from build123d import *

# Parameters (mm, degrees)
SKETCH_1_W          = 16
SKETCH_1_H          = 16
EXTRUDE_1_DEPTH     = 20
SKETCH_2_W          = 24
SKETCH_2_H          = 24
EXTRUDE_4_DEPTH     = 10
SKETCH_3_W          = 4
SKETCH_3_H          = 3
EXTRUDE_6_DEPTH     = 24
SKETCH_5_R          = 1.6
CUT_EXTRUDE_1_DEPTH = 24
CUT_EXTRUDE_2_DEPTH = 24


with BuildPart() as part:
    # 草图1 → 凸台-拉伸1 (new body)
    with BuildSketch(Plane(origin=(0, 0, 0), x_dir=(1, 0, 0), z_dir=(0, 1, 0))):
        Polygon((-4, 20), (-4, 16), (-4, -4), (16, -4), (20, -4), (20, 0), (20, 20), (0, 20), align=None)
        with Locations((8, 8)):
            Rectangle(SKETCH_1_W, SKETCH_1_H, mode=Mode.SUBTRACT)
    extrude(amount=-EXTRUDE_1_DEPTH)

    # 草图2 → 凸台-拉伸4 (add)
    with BuildSketch(Plane.XZ.offset(20)):
        with Locations((8, -8)):
            Rectangle(SKETCH_2_W, SKETCH_2_H)
    extrude(amount=EXTRUDE_4_DEPTH)

    # 草图3 → 凸台-拉伸6 (add)
    with BuildSketch(Plane.ZY.offset(4)):
        with Locations((10, -36.5)):
            Rectangle(SKETCH_3_W, SKETCH_3_H)
        with BuildLine():
            Line((4, -35), (4, -30))
            Line((4, -30), (-8.000000062, -30))
            ThreePointArc((-8.000000062, -30), (-2.343145773, -32.343145728), (0, -38))
            Line((0, -38), (8, -38))
            Line((8, -38), (8, -35))
            Line((8, -35), (4, -35))
        make_face()
        with BuildLine():
            ThreePointArc((-16, -38), (-13.656854272, -32.343145773), (-8.000000062, -30))
            Line((-8.000000062, -30), (-20, -30))
            Line((-20, -30), (-20, -35))
            Line((-20, -35), (-24, -35))
            Line((-24, -35), (-24, -38))
            Line((-24, -38), (-16, -38))
        make_face()
        with Locations((-26, -36.5)):
            Rectangle(SKETCH_3_W, SKETCH_3_H)
    extrude(amount=-EXTRUDE_6_DEPTH)

    # 草图5 → 切除-拉伸1 (cut)
    with BuildSketch(Plane.XZ.offset(38)):
        with Locations(Location((8, 9, 0), (0, 0, 270))):
            Circle(SKETCH_5_R)
        with Locations(Location((16, 9, 0), (0, 0, 270))):
            Circle(SKETCH_5_R)
        with Locations(Location((0, 9, 0), (0, 0, 90))):
            Circle(SKETCH_5_R)
        with Locations(Location((0, -25, 0), (0, 0, 270))):
            Circle(SKETCH_5_R)
        with Locations(Location((8, -25, 0), (0, 0, 270))):
            Circle(SKETCH_5_R)
        with Locations(Location((16, -25, 0), (0, 0, 270))):
            Circle(SKETCH_5_R)
    extrude(amount=-CUT_EXTRUDE_1_DEPTH, mode=Mode.SUBTRACT)

    # 草图6 → 切除-拉伸2 (cut)
    with BuildSketch(Plane.ZY.offset(4)):
        with BuildLine():
            Line((-20, -35), (-20, 0))
            Line((-20, 0), (4, 0))
            Line((4, 0), (4, -35))
            ThreePointArc((4, -35), (-8, -25.630683123), (-20, -35))
        make_face()
    extrude(amount=-CUT_EXTRUDE_2_DEPTH, mode=Mode.SUBTRACT)


solid = part.part
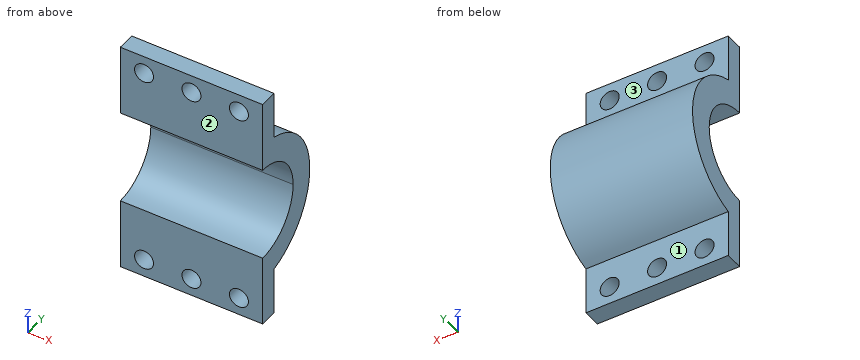
Work out the finished part from the listing and answer in its coordinate system (mm). Face numbers are marked on the shaded views. A direction names the side the tool comes from. Give positions to 0.01 mm unless a question says otherwise; leave off trailing zeros. Loops run counter-clockwise (first coordinate to the right, second up) from the corner with the lowest first, then second, coordinate; pieces in that order, holes last. Notation, with made-up numbers: M 61.25,33.5 L 86.25,33.5 A14 ccw 86.25,38.5 Z; hole C 28,20.25 d11. An arc over 180 degrees is marked long. Use CSV: the item, a comma, the result in double quotes.
1) Find section D-D on y = -34.5. Write down the section's boundary in (x, z), plus the area to 3 significant figures.
Answer:
outline,"M -4,-19.86 L 20,-19.86 L 20,-15.19 L -4,-15.19 Z; M -4,-0.81 L 20,-0.81 L 20,3.86 L -4,3.86 Z"
area,"224 mm^2"
2) Consider L1, parallel to X at y = -36.5, z = 9; L2, parallel to Z at x = -2, y = -33.75; L3, parallel to Z at x = 14.25, y = -36. Determine where each line is inside the solid, lowest interval first.
Answer:
L1,"-4 to -1.6, 1.6 to 6.4, 9.6 to 14.4, 17.6 to 20"
L2,"-19.62 to -14.78, -1.22 to 3.62"
L3,"-28 to -15.75, -0.25 to 12"
3) Find section B-B on x = 16. Write down the section's boundary in (y, z), plus the area to 3 significant figures.
Answer:
outline,"M -38,-28 L -35,-28 L -35,-26.6 L -38,-26.6 Z; M -38,-23.4 L -35,-23.4 L -35,-20 A12.37 ccw -35,4 L -35,7.4 L -38,7.4 L -38,0 A8 cw -38,-16 Z; M -38,10.6 L -35,10.6 L -35,12 L -38,12 Z"
area,"167 mm^2"
4) Given P1, Ø2, axis at x = 15, z = -12, coming from the -Y side (3 decimals); P2, Ø4, axis at x = 10, z = -15, coming from the +Y side; P3, Ø8, axis at x = 6, z = -22, coming from the +Y side, each flat-ended and moving along its own axis, determine where each tip first touches the part or whether it passes through.
Answer:
P1,"y = -31.755"
P2,"y = -26.69"
P3,"y = -30.72"
5) Find section C-C on y = -32.25. Write down the section's boundary in (x, z).
Answer:
outline,"M -4,-18.95 L 20,-18.95 L 20,-13.56 L -4,-13.56 Z; M -4,-2.44 L 20,-2.44 L 20,2.95 L -4,2.95 Z"
6) Which of the six approach directions +Z, -Z, +X, -X, +Y, -Y give full straight-line access (tool end or side, diameter ignored) to the marked faces 1, 2 and 3?
Answer:
face 1,"-Z, +X, -X, +Y"
face 2,"+Z, -Z, +X, -X, -Y"
face 3,"+Z, +X, -X, +Y"
7) Find section A-A on z = -25. Write down the section's boundary in (x, y).
Answer:
outline,"M -4,-38 L -1.6,-38 L -1.6,-35 L -4,-35 Z; M 1.6,-38 L 6.4,-38 L 6.4,-35 L 1.6,-35 Z; M 9.6,-38 L 14.4,-38 L 14.4,-35 L 9.6,-35 Z; M 17.6,-38 L 20,-38 L 20,-35 L 17.6,-35 Z"
